Check sheet for the modelled part. Datum: model origin and axes. Units: mm. A direction names the side the tool comes from. Round coordinates to 2 decimals unless told otherwise and drop trailing zeros. Order: outer loops, then holes, each group sorted by start corner. A loop starts at its lowest first (then second) coordinate and runs counter-clockwise, first axis right, second up.
```python
from build123d import *

# Parameters (mm, degrees)
SKETCH1_R               = 8.5
BOSS_EXTRUDE1_DEPTH     = 61
SKETCH2_W               = 39.5
SKETCH2_H               = 1
SKETCH3_W               = 27
SKETCH3_H               = 1.5
SKETCH4_W               = 1.1
SKETCH4_H               = 0.6
SKETCH5_W               = 1.1
SKETCH5_H               = 0.65
CUT_EXTRUDE1_DEPTH      = 63.173145328
CUT_EXTRUDE1_DEPTH_BACK = 63.173145328
SKETCH6_W               = 12
SKETCH6_H               = 12
CUT_EXTRUDE2_DEPTH      = 2.5


with BuildPart() as part:
    # Sketch1 → Boss-Extrude1 (new, symmetric)
    with BuildSketch(Plane.XY):
        with Locations(Location((0, 0, 0), (0, 0, 180))):
            Circle(SKETCH1_R)
    extrude(amount=BOSS_EXTRUDE1_DEPTH, both=True)

    # Sketch2 → Cut-Revolve1 (revolve, cut)
    with BuildSketch(Plane(origin=(0, 0, 0), x_dir=(0, 0, -1), z_dir=(1, 0, 0)), mode=Mode.PRIVATE) as cut_revolve1_sk:
        with Locations((41.25, 8)):
            Rectangle(SKETCH2_W, SKETCH2_H)
    cut_revolve1 = revolve(cut_revolve1_sk.sketch.rotate(Axis((0, 0, -67.1), (0, 0, 1)), 90), axis=Axis((0, 0, -67.1), (0, 0, 1)), mode=Mode.SUBTRACT)

    # Mirror1: Cut-Revolve1 across plane
    add(cut_revolve1.mirror(Plane.XY), mode=Mode.SUBTRACT)

    # Sketch3 → Cut-Revolve2 (revolve, cut)
    with BuildSketch(Plane(origin=(0, 0, 0), x_dir=(0, 0, -1), z_dir=(1, 0, 0)), mode=Mode.PRIVATE) as cut_revolve2_sk:
        with Locations((47.5, 6.75)):
            Rectangle(SKETCH3_W, SKETCH3_H)
    cut_revolve2 = revolve(cut_revolve2_sk.sketch.rotate(Axis((0, 0, -67.1), (0, 0, 1)), 90), axis=Axis((0, 0, -67.1), (0, 0, 1)), mode=Mode.SUBTRACT)

    # Mirror2: Cut-Revolve2 across plane
    add(cut_revolve2.mirror(Plane.XY), mode=Mode.SUBTRACT)

    # Sketch4 → Cut-Revolve3 (revolve, cut)
    with BuildSketch(Plane(origin=(0, 0, 0), x_dir=(0, 0, -1), z_dir=(1, 0, 0)), mode=Mode.PRIVATE) as cut_revolve3_sk:
        with Locations((30.95, 7.2)):
            Rectangle(SKETCH4_W, SKETCH4_H)
    cut_revolve3 = revolve(cut_revolve3_sk.sketch.rotate(Axis((0, 0, -67.1), (0, 0, 1)), 90), axis=Axis((0, 0, -67.1), (0, 0, 1)), mode=Mode.SUBTRACT)

    # Mirror3: Cut-Revolve3 across plane
    add(cut_revolve3.mirror(Plane.XY), mode=Mode.SUBTRACT)

    # Sketch5 → Cut-Revolve4 (revolve, cut)
    with BuildSketch(Plane(origin=(0, 0, 0), x_dir=(0, 0, -1), z_dir=(1, 0, 0)), mode=Mode.PRIVATE) as cut_revolve4_sk:
        with Locations((8.45, 8.175)):
            Rectangle(SKETCH5_W, SKETCH5_H)
    cut_revolve4 = revolve(cut_revolve4_sk.sketch.rotate(Axis((0, 0, -67.1), (0, 0, 1)), 90), axis=Axis((0, 0, -67.1), (0, 0, 1)), mode=Mode.SUBTRACT)

    # Mirror4: Cut-Revolve4 across plane
    add(cut_revolve4.mirror(Plane.XY), mode=Mode.SUBTRACT)

    # Sketch6 → Cut-Extrude1 (cut, two sides: drawn at the far end of the back side and taken through both)
    with BuildSketch(Plane(origin=(0, 0, 0), x_dir=(0, 0, -1), z_dir=(1, 0, 0)).offset(-CUT_EXTRUDE1_DEPTH_BACK)):
        with Locations((-55, 0)):
            Rectangle(SKETCH6_W, SKETCH6_H)
    extrude(amount=CUT_EXTRUDE1_DEPTH + CUT_EXTRUDE1_DEPTH_BACK, mode=Mode.SUBTRACT)

    # Sketch8 → Cut-Extrude2 (cut)
    with BuildSketch(Plane(origin=(0, 8.5, 0), x_dir=(1, 0, 0), z_dir=(0, 1, 0))):
        with BuildLine():
            Line((-2, -5.5), (-2, 5.5))
            ThreePointArc((-2, 5.5), (0, 7.5), (2, 5.5))
            Line((2, 5.5), (2, -5.5))
            ThreePointArc((2, -5.5), (0, -7.5), (-2, -5.5))
        make_face()
    extrude(amount=-CUT_EXTRUDE2_DEPTH, mode=Mode.SUBTRACT)


solid = part.part
```
Item 1: Sectioned sample at B-B (z = -16). Record the cut outline in (x, y), and give its area (3 significant figures).
Answer:
outline: circle Ø17 at (0, 0)
area: 227 mm2
Item 2: Access from +Z, -Z, +X, -X, +Y, -Y to the whole of each face (thin tool, end or side, straight path). Record for faces 4 (the cylindrical face through (1.107, -8.428, 0.111)), 5 (the cylindrical face through (-4.032, -6.324, -32.768)), 6 (the flat face through (2, -6, 34)), 7 (the cylindrical face through (0, 7.3, -7.5)), 8 (the flat face through (8, 2, -7.9)).
Answer:
face 4: +Z, -Z
face 5: -Z
face 6: +Z
face 7: +Y
face 8: none
Item 3: Go/stop test with flat-tipped pins: P1, Ø3, axis at x = 1, z = 2, coming from the +Y side; P2, Ø1.5, axis at x = -5.5, z = -12, coming from the -Y side; P3, Ø2, axis at y = -3, z = 22, coming from the +X side. Record where each tip stops, or that it passes through.
Answer:
P1: stops at y = 8.26
P2: stops at y = -7.05
P3: stops at x = 8.23
Item 4: Scan lines: line 1 along Z through (x, y) = (4.25, 6.75); line 2 along Z through (x, y) = (-7, -0.25); line 3 along Y through (x, z) = (6, 4). Record each from-to range of solid material in increasing order.
Answer:
line 1: z = -21.5 to -9, -7.9 to 7.9, 9 to 21.5
line 2: z = -34 to -31.5, -30.4 to 30.4, 31.5 to 34
line 3: y = -6.02 to 6.02
Item 5: Release check for a two-part mould opening along X. For faces 1 (the cylindrical face through (1.107, -8.428, -15.162)), 2 (the flat face through (2, 7, 0)), 3 (the flat face through (7, 2, -30.4)) record: released by +X, released by -X, zero draft, split by the parting line, or undercut.
Answer:
face 1: split by the parting line
face 2: undercut
face 3: zero draft
Item 6: Sectioned sample at A-A (z = -51). Record the cut outline in (x, y).
Answer:
outline: circle Ø12 at (0, 0)
